Work out the finished part from the listing and answer in its coordinate system (mm). A direction names the side the tool comes from. Give positions to 0.01 mm unless a question says otherwise; leave off trailing zeros. Write each loop counter-clockwise with the first axis right and the second up, starting at its lowest first coordinate (ties: lowest second). Pieces come first, ordered by that corner, then holes.
1) Find section A-A (y = -8.5). Determine the outline of the cut face in (x, z).
2) Find section D-D (x = 18.5). Determine the outline of the cut face in (y, z).
3) Find section B-B (x = 3.5). Determine the outline of the cut face in (y, z), plus the area to 3 significant figures.
4) Straight lines are drawn through the part: probe 1 along Y at (x, z) = (18.25, 1.05); probe 2 along X at (y, z) = (-10.5, 0.95); probe 3 along X at (y, z) = (8.25, 0.8). For each, find the intervals that lie inside material, in ascending order.
5) Find section C-C (z = 0.4). Determine the outline of the cut face in (x, y).
6) Given pin 1 Ø0.7 at (y, z) = (-4.5, 0.5) entering from -X; pin 2 Ø1 at (x, y) = (13, -8) entering from +Z; pin 3 Ø0.7 at (x, z) = (11.5, 1) entering from -Y, each flat-ended and moving along its own axis, determine where each tip first touches the part or whether it passes through.
7) A tool of negligible diameter and unlimited length cuts with its end or side. For faces 5 (the face through (18, -15.621, 1)), 6 (the face through (15.24, -8, 1)), 7 (the face through (19.71, -10, 1)), from which of +Z, -Z, +X, -X, +Y, -Y can it reach the whole face along a straight path? Write none if from no direction.
8) Determine the mould class of faces 1 (the face through (18.23, -13.08, 0.76)), 2 (the face through (11, 12.598, 1)), 3 (the face through (21.285, -2, 1)), 4 (the face through (3.02, 5.36, 0.76)) for opening direction X: pulls with the +X half, pulls with the -X half, needs draft (parallel to the pull), parting line crosses it, or undercut.
Autodesk Inventor part; units mm, degrees
ref_plane "YZ Plane" through (0, 0, 0) normal (1, 0, 0) x (0, 1, 0)
ref_plane "XZ Plane" through (0, 0, 0) normal (0, 1, 0) x (-1, 0, 0)
ref_plane "XY Plane" through (0, 0, 0) normal (0, 0, 1) x (1, 0, 0)
sketch "Sketch1" plane through (0, 0, 0) normal (0, 0, 1) x (1, 0, 0)
  line L0 (0, 0) -> (15.24, 0)
  line L1 (21.2852, 0) -> (21.2852, 12.5984)
  line L2 (21.2852, 12.5984) -> (0, 12.5984)
  line L3 (0, 12.5984) -> (0, 0)
  line L4 (15.24, 0) -> (15.24, -15.621)
  line L5 (15.24, -15.621) -> (21.2852, -15.621)
  line L6 (21.2852, -15.621) -> (21.2852, 0)
  line L7 (0, 0) -> (15.24, 0)
  dimension "d0" = 21.2852
  dimension "d1" = 12.5984
  dimension "d2" = 6.0452
  dimension "d3" = 15.621
extrude "Extrusion1" add sketch "Sketch1" along normal blind 1.4986
sketch "Sketch2" plane through (0, 0, 1.4986) normal (0, 0, 1) x (1, 0, 0)
  circle A0 centre (4.572, 6.5532) radius 1.9558
  line L0 (21.2852, 12.5984) -> (0, 12.5984)
  line L1 (0, 12.5984) -> (0, 0)
  circle A1 centre (18.2626, 6.5532) radius 1.9558
  dimension "d6" = 3.9116
  dimension "d7" = 6.0452
  dimension "d8" = 4.572
  dimension "d11" = 13.6906
extrude "Extrusion2" cut sketch "Sketch2" against normal blind 25.4
sketch "Sketch3" plane through (0, 0, 1.4986) normal (0, 0, 1) x (1, 0, 0)
  circle A0 centre (18.2626, -11.6332) radius 1.4478
  line L0 (15.24, -15.621) -> (21.2852, -15.621)
  line L1 (15.24, 0) -> (15.24, -15.621)
  circle A1 centre (18.2626, -7.6708) radius 1.4478
  line L2 (16.8148, -7.6708) -> (18.2626, -7.6708)
  line L3 (19.7104, -11.6332) -> (17.1196, -11.6332)
  point P0 (0, 0)
  dimension "d18" = 2.8956
  dimension "d19" = 3.9878
  dimension "d20" = 3.0226
  dimension "d26" = 3.9624
extrude "Extrusion4" cut sketch "Sketch3" against normal blind 25.4
sketch "Sketch6" plane through (0, 0, 1.4986) normal (0, 0, 1) x (1, 0, 0)
  circle A0 centre (18.2626, -7.6708) radius 1.4478
  circle A1 centre (18.2626, -11.6332) radius 1.4478
  line L0 (16.8148, -7.6708) -> (19.7104, -7.6708)
  line L1 (19.7104, -7.6708) -> (19.7104, -11.6332)
  line L2 (19.7104, -11.6332) -> (16.8148, -11.6332)
  line L3 (16.8148, -11.6332) -> (16.8148, -7.6708)
  point P0 (0, 0)
extrude "Extrusion5" cut sketch "Sketch6" against normal blind 25.4 contours L1 A1 L3 A0 | A0 L0 | L2 A1 picked at (18.2044, -8.1499) picked at (18.4337, -11.182)
equation "\"BendRadius\" = Thickness"
equation "\"BendReliefWidth\" = Thickness"
equation "\"BendReliefDepth\" = 0.5 * Thickness"
equation "\"CornerReliefSize\" = 4 * Thickness"
equation "\"MinimumRemnant\" = 2 * Thickness"
equation "\"TransitionRadius\" = BendRadius"
equation "\"JacobiRadiusSize\" = Thickness"
equation "\"GapSize\" = Thickness"
properties part number "dsub37bracket_redraw"
Results:
1. outline: (15.24, 0) - (16.81, 0) - (16.81, 1.5) - (15.24, 1.5) - close; (19.71, 0) - (21.29, 0) - (21.29, 1.5) - (19.71, 1.5) - close
2. outline: (-15.62, 0) - (-13.06, 0) - (-13.06, 1.5) - (-15.62, 1.5) - close; (-6.24, 0) - (4.61, 0) - (4.61, 1.5) - (-6.24, 1.5) - close; (8.49, 0) - (12.6, 0) - (12.6, 1.5) - (8.49, 1.5) - close
3. outline: (0, 0) - (4.92, 0) - (4.92, 1.5) - (0, 1.5) - close; (8.19, 0) - (12.6, 0) - (12.6, 1.5) - (8.19, 1.5) - close
3. area: 14.0 mm2
4. probe 1: y = -15.62 to -13.08, -6.22 to 4.6, 8.51 to 12.6
4. probe 2: x = 15.24 to 16.81, 19.71 to 21.29
4. probe 3: x = 0 to 3.6, 5.54 to 17.29, 19.24 to 21.29
5. outline: (0, 0) - (15.24, 0) - (15.24, -15.62) - (21.29, -15.62) - (21.29, 12.6) - (0, 12.6) - close; hole circle Ø3.91 at (4.57, 6.55); hole circle Ø3.91 at (18.26, 6.55); hole (16.81, -11.63) arc R1.45 ccw to (19.71, -11.63) - (19.71, -7.67) arc R1.45 ccw to (16.81, -7.67) - close
6. pin 1: stops at x = 15.24
6. pin 2: passes through
6. pin 3: stops at y = 0
7. face 5: +Z, -Z, +X, -X, -Y
7. face 6: +Z, -Z, -X, -Y
7. face 7: +Z, -Z
8. face 1: undercut
8. face 2: needs draft
8. face 3: pulls with the +X half
8. face 4: undercut
